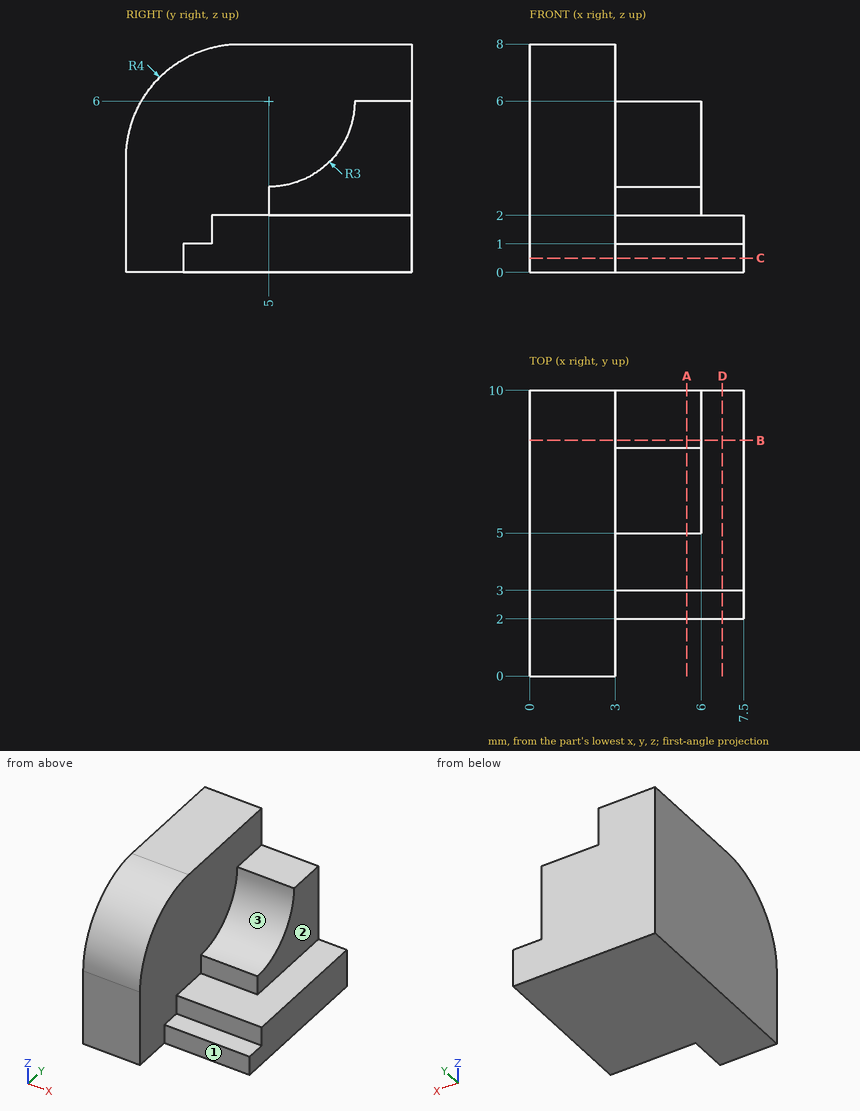
Drawing for the job (mm, zero at the part's lowest x, y, z). A direction names the side the tool comes from. Round coordinates to 2 decimals unless told otherwise and drop trailing zeros. Write each loop counter-clockwise with the first axis right and the second up, starting at its lowest first coordinate (ties: lowest second). Pieces come first, ordered by that corner, then holes. Notation, with made-up numbers: M 16,18.5 L 68,18.5 A26 ccw 68,51.5 Z; hole C 54,-17 d9. An arc over 180 degrees is marked long. Put each result on its own line as item: value.
Item 1: Cut at B-B (y = 8.25). List the corners of the cut face in (x, z), and give its area (3 significant figures).
Responses:
outline: M 0,0 L 7.5,0 L 7.5,2 L 6,2 L 6,6 L 3,6 L 3,8 L 0,8 Z
area: 45.0 mm²
Item 2: Tool access for the marked faces 1, 2 and 3: list every direction of +Z, -Z, +X, -X, +Y, -Y with a clear straight run to the whole face (end or side of a thin tool).
Responses:
face 1: +Z, -Z, +X, -Y
face 2: +Z, +X, +Y, -Y
face 3: +Z, +X, -Y
Item 3: Cut at C-C (z = 0.5). List the corners of the cut face in (x, y), and give its area (3 significant figures).
Responses:
outline: M 0,0 L 3,0 L 3,2 L 7.5,2 L 7.5,10 L 0,10 Z
area: 66.0 mm²
Item 4: Cut at D-D (x = 6.75). List the corners of the cut face in (y, z), and give its area (3 significant figures).
Responses:
outline: M 2,0 L 10,0 L 10,2 L 3,2 L 3,1 L 2,1 Z
area: 15.0 mm²
Item 5: Cut at A-A (x = 5.5). List the corners of the cut face in (y, z), and give its area (3 significant figures).
Responses:
outline: M 2,0 L 10,0 L 10,6 L 8,6 A3 cw 5,3 L 5,2 L 3,2 L 3,1 L 2,1 Z
area: 27.9 mm²
Item 6: Probe L1, parallel to X at y = 0.5, z = 3; L2, parallel to Z at x = 3.5, y = 4.25; L3, parallel to Y at x = 3.75, z = 2.5. List the from-to ranges inside material, lowest first. Write a range as from..to.
Responses:
L1: 0..3
L2: 0..2
L3: 5..10
Item 7: Flat gauge pins, fed straight in: P1, Ø3, axis at y = 6.5, z = 4, coming from the +X side; P2, Ø0.5, axis at x = 5, z = 2.5, coming from the -Y side; P3, Ø1.1, axis at x = 4.5, z = 1.5, coming from the -Y side. Where does each tip first touch, or does it go through?
Responses:
P1: x = 6
P2: y = 5
P3: y = 2
